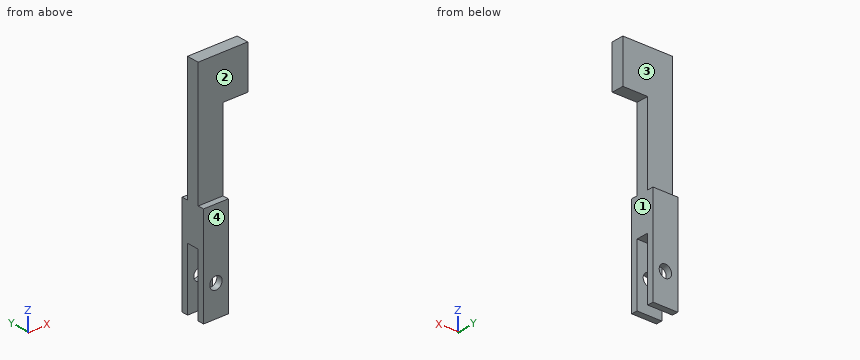
from build123d import *

# Parameters (mm, degrees)
F1_DEPTH = 20
F2_W     = 40
F2_H     = 5
F3_DEPTH = 100
F4_W     = 20
F4_H     = 10
F5_DEPTH = 50
F6_R     = 5
F7_DEPTH = 20.001


with BuildPart() as f1:
    # F0 (on Front) → F1 (new body)
    with BuildSketch(Plane.XZ):
        Polygon((-19.255103, 180), (-19.255103, 0), (0.744897, 0), (0.744897, 145), (20.744897, 145), (20.744897, 180), align=None)
    extrude(amount=-F1_DEPTH)

    # F2 (on face) → F3 (cut)
    with BuildSketch(Plane.XY.offset(180)):
        with Locations((0.744897, 17.5)):
            Rectangle(F2_W, F2_H)
        with Locations((0.744897, 2.5)):
            Rectangle(F2_W, F2_H)
    extrude(amount=-F3_DEPTH, mode=Mode.SUBTRACT)

    # F4 (on face) → F5 (cut)
    with BuildSketch(Plane(origin=(0, 0, 0), x_dir=(1, 0, 0), z_dir=(0, 0, -1))):
        with Locations((-9.255103, -10)):
            Rectangle(F4_W, F4_H)
    extrude(amount=-F5_DEPTH, mode=Mode.SUBTRACT)

    # F6 (on face) → F7 (cut, through all)
    with BuildSketch(Plane.XZ):
        with Locations((-9.255103, 25)):
            Circle(F6_R)
    extrude(amount=-F7_DEPTH, mode=Mode.SUBTRACT)


solid = f1.part
The listing builds one solid part. Answer for the finished solid, in the listing's coordinates (mm). Face numbers are marked on the shaded views. A direction names the side the tool comes from. Give positions to 0.01 mm unless a question says otherwise; leave off trailing zeros. Write each loop counter-clockwise with the first axis right and the second up, starting at its lowest first coordinate (ties: lowest second). Pieces come first, ordered by that corner, then holes.
1) Section A-A (z = 25) is taken. Write down the section's boundary in (x, y).
2) Section D-D (x = -11) is taken. Write down the section's boundary in (y, z), and give its area (3 significant figures).
3) Section B-B (x = -2.5) is taken. Write down the section's boundary in (y, z).
4) Given P1, Ø10, axis at x = -7.5, z = 13.5, coming from the -Y side; P2, Ø1, axis at x = -4, y = 14, coming from the -Z side; P3, Ø12, axis at x = -1.5, z = 127, coming from the +Y side; P4, Ø1.5, axis at x = -13.5, y = 2.5, coming from the +Z side, each flat-ended and moving along its own axis, determine where each tip first touches the part or whether it passes through.
5) Find the intervals of material crossed by L1, parallel to Z at x = 2.5, y = 10.75; L2, parallel to Z at x = 0, y = 7; L3, parallel to X at y = 5.75, z = 71.5, in increasing order.
6) Section C-C (y = 2.5) is taken. Write down the section's boundary in (x, z), and give its area (3 significant figures).
7) A tool of negligible diameter and unlimited length cuts with its end or side. For the marked faces 1, 2, 3 and 4, from which of +Z, -Z, +X, -X, +Y, -Y can it reach the whole face along a straight path? Write none if from no direction.
Response:
1. outline: (-19.26, 0) - (-14.26, 0) - (-14.26, 5) - (-19.26, 5) - close; (-19.26, 15) - (-14.26, 15) - (-14.26, 20) - (-19.26, 20) - close; (-4.26, 0) - (0.74, 0) - (0.74, 5) - (-4.26, 5) - close; (-4.26, 15) - (0.74, 15) - (0.74, 20) - (-4.26, 20) - close
2. outline: (0, 0) - (5, 0) - (5, 20.31) - (0, 20.31) - close; (0, 29.69) - (5, 29.69) - (5, 50) - (15, 50) - (15, 29.69) - (20, 29.69) - (20, 80) - (15, 80) - (15, 180) - (5, 180) - (5, 80) - (0, 80) - close; (15, 0) - (20, 0) - (20, 20.31) - (15, 20.31) - close
2. area: 2,010 mm2
3. outline: (0, 0) - (5, 0) - (5, 50) - (15, 50) - (15, 0) - (20, 0) - (20, 80) - (15, 80) - (15, 180) - (5, 180) - (5, 80) - (0, 80) - close
4. P1: stops at y = 0
4. P2: stops at z = 50
4. P3: stops at y = 15
4. P4: stops at z = 80
5. L1: z = 145 to 180
5. L2: z = 50 to 180
5. L3: x = -19.26 to 0.74
6. outline: (-19.26, 0) - (0.74, 0) - (0.74, 80) - (-19.26, 80) - close; hole circle Ø10 at (-9.26, 25)
6. area: 1,520 mm2
7. face 1: -Z, +X, +Y, -Y
7. face 2: +Z, +X, -X, -Y
7. face 3: +Z, +X, -X, +Y
7. face 4: +Z, -Z, +X, -X, -Y
